CAD build for the part. Positions are in the model's coordinates, mm. Coordinates: 2 decimals unless noted, no trailing zeros. Order: outer loops, then holes, each group sorted by start corner. A loop starts at its lowest first (then second) coordinate and runs counter-clockwise, first axis right, second up. Notation, with made-up numbers: (-10, 78.25) - (47, 78.25) arc R32 ccw to (47, 115.25) - close; hole circle Ø5 at (58, 26.25). An arc over 180 degrees is marked (long way). Use one line per item in the form item = value.
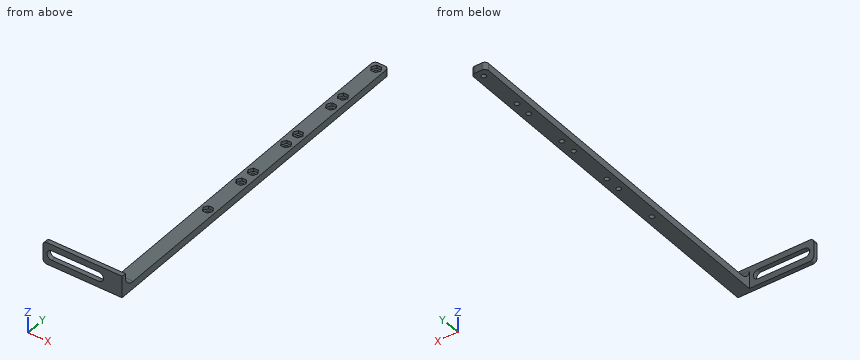
```python
from build123d import *

# Parameters (mm, degrees)
PAD_DEPTH                    = 5
POCKET_DEPTH                 = 2.15
SKETCH002_R                  = 1.6
HOLE_DEPTH                   = 501.352755
POCKET_LINEARPATTERN_2_DEPTH = 2.15
SKETCH002_LINEARPATTERN_2_R  = 1.6
HOLE_LINEARPATTERN_2_DEPTH   = 501.352755
LINEARPATTERN001_COUNT       = 4
LINEARPATTERN001_PITCH       = 42
PAD001_DEPTH                 = 3
POCKET001_DEPTH              = 3.001
PAD002_DEPTH                 = 10


with BuildPart() as part:
    # Sketch → Pad (new body)
    with BuildSketch(Plane.XY):
        with BuildLine():
            Line((0, 5), (-2.5, 5))
            ThreePointArc((-2.5, 5), (-4.267767, 4.267767), (-5, 2.5))
            Line((-5, 2.5), (-5, -244))
            Line((-5, -244), (0, -244))
            Line((0, -244), (0, 5))
        make_face()
    pad = extrude(amount=PAD_DEPTH)

    # Mirrored: Pad across Sketch V_Axis
    add(pad.mirror(Plane(origin=(0, 0, 0), x_dir=(0, 0, 1), z_dir=(1, 0, 0))))

    # Sketch001 (on Face5 of Mirrored) → Pocket (cut)
    with BuildSketch(Plane.XY.offset(5)):
        Polygon((3.348632, 0), (1.674316, 2.9), (-1.674316, 2.9), (-3.348632, 0), (-1.674316, -2.9), (1.674316, -2.9), align=None)
    pocket = extrude(amount=-POCKET_DEPTH, mode=Mode.SUBTRACT)

    # Sketch002 (on Face19 of Pocket) → Hole (cut, through all)
    with BuildSketch(Plane.XY.offset(2.85)):
        Circle(SKETCH002_R)
    hole = extrude(amount=-HOLE_DEPTH, mode=Mode.SUBTRACT)

    # Sketch001 LinearPattern 2 → Pocket LinearPattern 2 (cut)
    with BuildSketch(Plane(origin=(0, -31, 5), x_dir=(1, 0, 0), z_dir=(0, 0, 1))):
        Polygon((3.348632, 0), (1.674316, 2.9), (-1.674316, 2.9), (-3.348632, 0), (-1.674316, -2.9), (1.674316, -2.9), align=None)
    pocket_linearpattern_2 = extrude(amount=-POCKET_LINEARPATTERN_2_DEPTH, mode=Mode.SUBTRACT)

    # Sketch002 LinearPattern 2 → Hole LinearPattern 2 (cut, through all)
    with BuildSketch(Plane(origin=(0, -31, 2.85), x_dir=(1, 0, 0), z_dir=(0, 0, 1))):
        Circle(SKETCH002_LINEARPATTERN_2_R)
    hole_linearpattern_2 = extrude(amount=-HOLE_LINEARPATTERN_2_DEPTH, mode=Mode.SUBTRACT)

    # LinearPattern001: Pocket, Hole, Pocket LinearPattern 2, Hole LinearPattern 2 ×4
    with Locations(*[(0, -i * LINEARPATTERN001_PITCH, 0) for i in range(1, LINEARPATTERN001_COUNT)]):
        add(pocket, mode=Mode.SUBTRACT)
        add(hole, mode=Mode.SUBTRACT)
        add(pocket_linearpattern_2, mode=Mode.SUBTRACT)
        add(hole_linearpattern_2, mode=Mode.SUBTRACT)

    # Sketch004 (on Face15 of MultiTransform) → Pad001 (join)
    with BuildSketch(Plane.XZ.offset(244)):
        with BuildLine():
            Line((5, 0), (-46.5, 0))
            ThreePointArc((-49, 2.5), (-48.267767, 0.732233), (-46.5, 0))
            Line((-49, 2.5), (-49, 7.5))
            Line((-49, 7.5), (5, 7.5))
            Line((5, 7.5), (5, 0))
        make_face()
    pad001 = extrude(amount=-PAD001_DEPTH)

    # Mirrored001: Pad001 across face of Pad001
    add(pad001.mirror(Plane(origin=(-22, -242.5, 7.5), x_dir=(1, 0, 0), z_dir=(0, 0, 1))))

    # Sketch005 (on Face51 of Mirrored001) → Pocket001 (cut, through all)
    with BuildSketch(Plane(origin=(0, -241, 0), x_dir=(-1, 0, 0), z_dir=(0, 1, 0))):
        with BuildLine():
            ThreePointArc((43, 4.235), (46.265, 7.5), (43, 10.765))
            Line((43, 10.765), (11, 10.765))
            ThreePointArc((11, 10.765), (7.735, 7.5), (11, 4.235))
            Line((43, 4.235), (11, 4.235))
        make_face()
    extrude(amount=-POCKET001_DEPTH, mode=Mode.SUBTRACT)

    # Sketch007 (on Face52 of Pocket001) → Pad002 (join)
    with BuildSketch(Plane.YZ.offset(5)):
        with BuildLine():
            Line((-241, 5), (-233.499977, 5))
            ThreePointArc((-241, 12.500001), (-238.803293, 7.196691), (-233.499977, 5))
            Line((-241, 5), (-241, 12.500001))
        make_face()
    extrude(amount=-PAD002_DEPTH)


solid = part.part
```
Item 1: Cut at C-C, the plane y = -163. Write the cut outline in (x, z), plus the area to 3 significant figures.
Derived:
outline = (-5, 0) - (5, 0) - (5, 5) - (-5, 5) - close
area = 50.0 mm²
Item 2: Drill centre lines: line 1 (X direction, y = -157, z = 1.8); line 2 (Y direction, x = -34.5, z = 13); line 3 (X direction, y = -155.5, z = 4.5). Where is each one in solid material? Low to high. Write a range as [from, to].
Derived:
line_1 = [-5, -1.6], [1.6, 5]
line_2 = [-244, -241]
line_3 = [-5, -2.48], [2.48, 5]
Item 3: Cut at A-A, the plane x = -25.5. Write the cut outline in (y, z) (3 decimals), plus the area to 3 significant figures.
Derived:
outline = (-244, 0) - (-241, 0) - (-241, 4.235) - (-244, 4.235) - close; (-244, 10.765) - (-241, 10.765) - (-241, 15) - (-244, 15) - close
area = 25.4 mm²
Item 4: Drop flat-ended pins along their axis: pin 1 (1.5 mm diameter, centred on y = -206, z = 3, fed in from -X); pin 2 (2.5 mm diameter, centred on x = 0, y = -157, fed in from -Z); pin 3 (6.5 mm diameter, centred on x = -1.5, y = -30.5, fed in from +Z); pin 4 (4 mm diameter, centred on x = 0, y = -115, fed in from +Z). Give the stop position or say it passes through.
Derived:
pin_1 = -5
pin_2 = through
pin_3 = 5
pin_4 = 2.85
Item 5: Cut at B-B, the plane z = 7.75. Write the cut outline in (x, y).
Derived:
outline = (-49, -244) - (-46.26, -244) - (-46.26, -241) - (-49, -241) - close; (-7.74, -244) - (5, -244) - (5, -239.3) - (-5, -239.3) - (-5, -241) - (-7.74, -241) - close
